CAD build for the part. Positions are in the model's coordinates, mm. Give positions to 0.01 mm unless a question says otherwise; leave off trailing zeros. Loops run counter-clockwise (first coordinate to the right, second up) from the corner with the lowest first, then second, coordinate; pieces in that order, holes last. Notation, with made-up numbers: M 78.25,42.25 L 92.25,42.25 A16 cw 92.25,52.25 Z; hole C -6,7.25 d6. An arc over 180 degrees is marked long. Answer as CSV lines item,"result".
from build123d import *

# Parameters (mm, degrees)
BOSS_EXTRUDE1_DEPTH = 87
SKETCH3_R           = 0.5
BOSS_EXTRUDE2_DEPTH = 10


with BuildPart() as part:
    # Sketch1 → Boss-Extrude1 (new body)
    with BuildSketch(Plane(origin=(0, 0, 0), x_dir=(1, 0, 0), z_dir=(0, 1, 0))):
        with BuildLine():
            Line((-16.634262286, -97.085278586), (-16.634262286, -98.606801582))
            ThreePointArc((-16.634262286, -98.606801582), (0, 100), (16.634262286, -98.606801582))
            Line((16.634262286, -98.606801582), (16.634262286, -97.085278586))
            ThreePointArc((16.634262286, -97.085278586), (0, 98.5), (-16.634262286, -97.085278586))
        make_face()
    extrude(amount=BOSS_EXTRUDE1_DEPTH)

    # Sketch3 → Boss-Extrude2 (add)
    # profile 1 of 3: a face of its own
    with BuildSketch(Plane(origin=(0, 87, 0), x_dir=(1, 0, 0), z_dir=(0, 1, 0))):
        with BuildLine():
            Line((-102.5, -2.5), (-99.33644021, -4.400913329))
            Line((-99.33644021, -4.400913329), (-99.185511668, 3.770789156))
            Line((-99.185511668, 3.770789156), (-102.5, 2.5))
            ThreePointArc((-102.5, 2.5), (-105, 0), (-102.5, -2.5))
        make_face()
        with Locations(Location((-102.5, 0, 0), (0, 0, 270))):
            Circle(SKETCH3_R, mode=Mode.SUBTRACT)
    # profile 2 of 3: a face of its own
    with BuildSketch(Plane(origin=(0, 87, 0), x_dir=(1, 0, 0), z_dir=(0, 1, 0))):
        with BuildLine():
            Line((-2.5, 102.5), (-4.400913329, 99.33644021))
            Line((-4.400913329, 99.33644021), (3.770789156, 99.185511668))
            Line((3.770789156, 99.185511668), (2.5, 102.5))
            ThreePointArc((2.5, 102.5), (0, 105), (-2.5, 102.5))
        make_face()
        with Locations(Location((0, 102.5, 0), (0, 0, 270))):
            Circle(SKETCH3_R, mode=Mode.SUBTRACT)
    # profile 3 of 3: a face of its own
    with BuildSketch(Plane(origin=(0, 87, 0), x_dir=(1, 0, 0), z_dir=(0, 1, 0))):
        with BuildLine():
            Line((102.5, 2.5), (99.33644021, 4.400913329))
            Line((99.33644021, 4.400913329), (99.185511668, -3.770789156))
            Line((99.185511668, -3.770789156), (102.5, -2.5))
            ThreePointArc((102.5, -2.5), (105, 0), (102.5, 2.5))
        make_face()
        with Locations(Location((102.5, 0, 0), (0, 0, 270))):
            Circle(SKETCH3_R, mode=Mode.SUBTRACT)
    extrude(amount=-BOSS_EXTRUDE2_DEPTH)


solid = part.part
1) Flat gauge pins, fed straight in: pin 1 (2 mm diameter, centred on x = 37, y = 42, fed in from +Z); pin 2 (2.5 mm diameter, centred on x = 0, z = -103, fed in from -Y); pin 3 (5 mm diameter, centred on y = 71.5, z = -79.5, fed in from -X); pin 4 (12 mm diameter, centred on x = -81.5, z = 71, fed in from +Y). Where does each tip first touch, or does it go through?
Answer below:
pin 1,"stops at z = 93.3"
pin 2,"stops at y = 77"
pin 3,"stops at x = -63.8"
pin 4,"passes through"
2) Band-saw the part on A-A on z = -69.5. Give the cut face in (x, y).
Answer below:
outline,"M -71.9,0 L -69.8,0 L -69.8,87 L -71.9,87 Z; M 69.8,0 L 71.9,0 L 71.9,87 L 69.8,87 Z"
3) Band-saw the part on D-D on x = -8. Give the cut face in (y, z), and give its area (3 significant figures).
Answer below:
outline,"M 0,-99.68 L 87,-99.68 L 87,-98.17 L 0,-98.17 Z"
area,"131 mm^2"
4) Band-saw the part on B-B on x = -52.5. Give the cut face in (y, z), and give its area (3 significant figures).
Answer below:
outline,"M 0,-85.11 L 87,-85.11 L 87,-83.34 L 0,-83.34 Z; M 0,83.34 L 87,83.34 L 87,85.11 L 0,85.11 Z"
area,"308 mm^2"
5) Mould opens along Z. For faces 1 (the face through (0, 82, -105)), 2 (the face through (-59, 0, 80)), 3 (the face through (4.097, 42.891, -98.415)), 4 (the face through (105, 82, 0)) say: +Z half, -Z half, draft (parallel to the pull), parting line (faces both ways), or undercut.
Answer below:
face 1,"-Z half"
face 2,"draft"
face 3,"undercut"
face 4,"parting line"
6) Drill centre lines: line 1 (X direction, y = 83, z = 0); line 2 (Z direction, x = 102.5, y = 82); line 3 (X direction, y = 33.5, z = -87.5). Where is each one in solid material? Low to high. Write a range as from..to.
Answer below:
line 1,"x = -105..-103, -102..-98.5, 98.5..102, 103..105"
line 2,"z = -2.5..-0.5, 0.5..2.5"
line 3,"x = -48.41..-45.23, 45.23..48.41"
7) Band-saw the part on C-C on y = 55. Give the cut face in (x, z).
Answer below:
outline,"M -16.63,97.09 L -16.63,98.61 A100 ccw long 16.63,98.61 L 16.63,97.09 A98.5 cw long Z"
